from build123d import *

# Parameters (mm, degrees)
F1_DEPTH = 6.0198
F3_DEPTH = 6.0198
F4_R     = 7.62
F5_R     = 1.27
F6_R     = 2.4765
F7_DEPTH = 6.0198


with BuildPart() as f1:
    # F0 (on Top) → F1 (new body)
    with BuildSketch(Plane.XY):
        with BuildLine():
            ThreePointArc((-5.588, -10.4775), (0, 11.8745), (5.588, -10.4775))
            Line((5.588, -10.4775), (5.588, -17.0815))
            Line((5.588, -17.0815), (19.1516, -17.0815))
            Line((19.1516, -17.0815), (19.1516, 21.4503))
            Line((19.1516, 21.4503), (-6.5024, 38.3413))
            ThreePointArc((-6.5024, 38.3413), (-15.638779, 32.001463), (-19.1516, 21.4503))
            Line((-19.1516, 21.4503), (-19.1516, -17.0815))
            Line((-19.1516, -17.0815), (-5.588, -17.0815))
            Line((-5.588, -17.0815), (-5.588, -10.4775))
        make_face()
    extrude(amount=F1_DEPTH)

    # F2 (on face) → F3 (cut, through all)
    with BuildSketch(Plane.XY.offset(6.0198)):
        with BuildLine():
            ThreePointArc((-6.026316, 32.343552), (-11.145726, 27.932464), (-13.0556, 21.4503))
            ThreePointArc((-13.0556, 21.4503), (-10.5156, 18.9103), (-7.9756, 21.4503))
            ThreePointArc((-7.9756, 21.4503), (-6.877265, 25.178077), (-3.933183, 27.714816))
            ThreePointArc((-3.933183, 27.714816), (-2.665381, 31.07575), (-6.026316, 32.343552))
        make_face()
    extrude(amount=-F3_DEPTH, mode=Mode.SUBTRACT)

    # F4
    f4_edges = [f1.edges().sort_by_distance(p)[0] for p in [
        (-6.5024, 38.3413, 3.0099),
        (19.1516, 21.4503, 3.0099),
    ]]
    fillet(f4_edges, radius=F4_R)

    # F5
    f5_edges = [f1.edges().sort_by_distance(p)[0] for p in [
        (-19.1516, -17.0815, 3.0099),
        (-5.588, -17.0815, 3.0099),
        (5.588, -17.0815, 3.0099),
        (19.1516, -17.0815, 3.0099),
        (5.588, -10.4775, 3.0099),
        (-5.588, -10.4775, 3.0099),
    ]]
    fillet(f5_edges, radius=F5_R)

    # F6 (on face) → F7 (cut, through all)
    with BuildSketch(Plane.XY.offset(6.0198)):
        with Locations((13.208606, 18.247754)):
            Circle(F6_R)
        with Locations((-12.3698, -13.51257)):
            Circle(F6_R)
        with Locations((12.3698, -13.51257)):
            Circle(F6_R)
    extrude(amount=-F7_DEPTH, mode=Mode.SUBTRACT)


solid = f1.part
Input: part model. Units: mm. Frame: model coordinates. A direction names the side the tool comes from. Coordinates: 2 decimals unless noted, no trailing zeros. Loops run counter-clockwise (first coordinate to the right, second up) from the corner with the lowest first, then second, coordinate; pieces in that order, holes last. Notation, with made-up numbers: (57.25, 66.25) - (94.25, 66.25) arc R19 cw to (94.25, 77.25) - close; hole circle Ø8 at (1, 24). An arc over 180 degrees is marked (long way). Answer in a Markdown table with one row per item. Add a question column.
Item 1: Access query for faces 5 (the cylindrical face through (-10.57, 18.91, 3.05)), 6 (the flat face through (19.152, 1, 3)), 7 (the flat face through (-5.588, -14, 3)). Directions: +Z, -Z, +X, -X, +Y, -Y. A direction counts if a zero-diameter tool reaches every point of the face in a straight line with its end or side. Return the directions, or none.
Item 2: Section query A-A on y = 0. Return the cut outline in (x, z).
Item 3: Section query B-B on z = 2.75. Return the cut outline in (x, y).
Item 4: Contact query for flat-ended pins moving along their axis: P1, Ø2, axis at y = 24.5, z = 5, coming from the -X side; P2, Ø3, axis at x = 15, z = 1.5, coming from the +Y side. Output: stop coordinate, or through.
Item 5: Mould query, pull axis Y, two halves, no side actions, for faces 1 (the cylindrical face through (-14.335, -15.019, 3.052)), 2 (the flat face through (5.588, -13, 3)), 3 (the cylindrical face through (18.79, -16.7, 3.05)), 4 (the cylindrical face through (-5.755, -10.585, 3.052)). Classes: released by +Y, released by -Y, zero draft, split by the parting line, or undercut.
Item 6: Line query: line 1 along X through (y, z) = (-13, 2.75); line 2 along Y through (x, z) = (-9, 0.75); line 3 along X through (y, z) = (-12, 1.75). Output: solid intervals per line, ascending. Write a range as [from, to].
Item 7: Section query C-C on y = 10. Return the cut outline in (x, z).
Item 8: Section query D-D on x = -15.5. Return the cut outline in (y, z), then the cut area to 3 significant figures.
Recorded:
| question | item | result |
|---|---|---|
| 1 | face 5 | +Z, -Z |
| 1 | face 6 | +Z, -Z, +X, +Y, -Y |
| 1 | face 7 | +Z, -Z, -Y |
| 2 | outline | (-19.15, 0) - (-11.87, 0) - (-11.87, 6.02) - (-19.15, 6.02) - close; (11.87, 0) - (19.15, 0) - (19.15, 6.02) - (11.87, 6.02) - close |
| 3 | outline | (-19.15, -15.81) arc R1.27 ccw to (-17.88, -17.08) - (-6.86, -17.08) arc R1.27 ccw to (-5.59, -15.81) - (-5.59, -11.21) arc R1.27 ccw to (-6.2, -10.13) arc R11.87 cw (long way) to (6.2, -10.13) arc R1.27 ccw to (5.59, -11.21) - (5.59, -15.81) arc R1.27 ccw to (6.86, -17.08) - (17.88, -17.08) arc R1.27 ccw to (19.15, -15.81) - (19.15, 17.34) arc R7.62 ccw to (15.72, 23.71) - (-3.01, 36.04) arc R7.62 ccw to (-11.52, 35.96) arc R17.6 ccw to (-19.15, 21.45) - close; hole circle Ø4.95 at (-12.37, -13.51); hole (-13.06, 21.45) arc R2.54 ccw to (-7.98, 21.45) arc R6.88 cw to (-3.93, 27.71) arc R2.54 ccw to (-6.03, 32.34) arc R11.96 ccw to start; hole circle Ø4.95 at (12.37, -13.51); hole circle Ø4.95 at (13.21, 18.25) |
| 4 | P1 | x = -19.03 |
| 4 | P2 | y = 25.17 |
| 5 | face 1 | undercut |
| 5 | face 2 | zero draft |
| 5 | face 3 | released by -Y |
| 5 | face 4 | undercut |
| 6 | line 1 | [-19.15, -14.79], [-9.95, -5.59], [5.59, 9.95], [14.79, 19.15] |
| 6 | line 2 | [-17.08, -7.75], [7.75, 19.41], [30.42, 37.08] |
| 6 | line 3 | [-19.15, -14.33], [-10.41, -5.59], [5.59, 10.41], [14.33, 19.15] |
| 7 | outline | (-19.15, 0) - (-6.4, 0) - (-6.4, 6.02) - (-19.15, 6.02) - close; (6.4, 0) - (19.15, 0) - (19.15, 6.02) - (6.4, 6.02) - close |
| 8 | outline | (-17.08, 0) - (32.18, 0) - (32.18, 6.02) - (-17.08, 6.02) - close |
| 8 | area | 297 mm^2 |
